```python
from build123d import *

# Parameters (mm, degrees)
F0_W      = 12.7
F0_H      = 50.8
F1_DEPTH  = 11.0998
F3_DEPTH  = 5.08
F3_TAPER  = 3
F4_W      = 12.7
F4_H      = 19.05
F5_DEPTH  = 47.0916
F6_W      = 6.35
F6_H      = 19.05
F7_DEPTH  = 126.7968
F8_W      = 12.7
F8_H      = 19.05
F9_DEPTH  = 40.7416
F10_W     = 12.7
F10_H     = 50.8
F11_DEPTH = 11.0998
F13_DEPTH = 5.334
F13_TAPER = 3
F14_W     = 25.4
F14_H     = 76.2
F15_DEPTH = 12.7
F16_W     = 25.4
F16_H     = 76.2
F17_DEPTH = 12.7
F18_R     = 3.96875
F19_DEPTH = 139.4978
F20_R     = 2.54
F21_DEPTH = 16.4348001
F22_R     = 2.54
F23_DEPTH = 58.1924
F24_R     = 3.81
F25_DEPTH = 45.4914
F26_R     = 6.35


with BuildPart() as f1:
    # F0 (on Right) → F1 (new body)
    with BuildSketch(Plane.YZ):
        with Locations((6.35, 25.4)):
            Rectangle(F0_W, F0_H)
    extrude(amount=F1_DEPTH)

    # F2 (on face) → F3 (join)
    with BuildSketch(Plane.YZ.offset(11.0998)):
        Polygon((4.191, 34.3605023065), (8.509, 34.3605023065), (10.668, 38.1), (8.509, 41.8394976935), (4.191, 41.8394976935), (2.032, 38.1), align=None)
    extrude(amount=F3_DEPTH, taper=F3_TAPER)

    # F4 (on face) → F5 (join)
    with BuildSketch(Plane(origin=(0, 0, 0), x_dir=(0, -1, 0), z_dir=(-1, 0, 0))):
        with Locations((-6.35, 9.525)):
            Rectangle(F4_W, F4_H)
    extrude(amount=F5_DEPTH)

    # F6 (on face) → F7 (join)
    with BuildSketch(Plane.XZ):
        with Locations((-43.9166, 9.525)):
            Rectangle(F6_W, F6_H)
    extrude(amount=F7_DEPTH)

    # F8 (on face) → F9 (join, through all)
    with BuildSketch(Plane.YZ.offset(-40.7416)):
        with Locations((-120.4468, 9.525)):
            Rectangle(F8_W, F8_H)
    extrude(amount=F9_DEPTH)

    # F10 (on face) → F11 (join)
    with BuildSketch(Plane.YZ):
        with Locations((-120.4468, 25.4)):
            Rectangle(F10_W, F10_H)
    extrude(amount=F11_DEPTH)

    # F12 (on face) → F13 (join)
    with BuildSketch(Plane.YZ.offset(11.0998)):
        Polygon((-118.2878, 41.8394976935), (-122.6058, 41.8394976935), (-124.7648, 38.1), (-122.6058, 34.3605023065), (-118.2878, 34.3605023065), (-116.1288, 38.1), align=None)
    extrude(amount=F13_DEPTH, taper=F13_TAPER)

    # F14 (on face) → F15 (join, through all)
    with BuildSketch(Plane(origin=(0, 12.7, 0), x_dir=(-1, 0, 0), z_dir=(0, 1, 0))):
        with Locations((34.3916, 38.1)):
            Rectangle(F14_W, F14_H)
    extrude(amount=-F15_DEPTH)

    # F16 (on face) → F17 (join, through all)
    with BuildSketch(Plane.XZ.offset(126.7968)):
        with Locations((-34.3916, 38.1)):
            Rectangle(F16_W, F16_H)
    extrude(amount=-F17_DEPTH)

    # F18 (on face) → F19 (cut, through all)
    with BuildSketch(Plane(origin=(0, 12.7, 0), x_dir=(-1, 0, 0), z_dir=(0, 1, 0))):
        with Locations((28.4226, 20.9296)):
            Circle(F18_R)
        with Locations((28.4226, 55.3466)):
            Circle(F18_R)
    extrude(amount=-F19_DEPTH, mode=Mode.SUBTRACT)

    # F20 (on face) → F21 (cut, through all)
    with BuildSketch(Plane(origin=(0, 0, 0), x_dir=(0, -1, 0), z_dir=(-1, 0, 0))):
        with Locations((-6.35, 6.35)):
            Circle(F20_R)
    extrude(amount=-F21_DEPTH, mode=Mode.SUBTRACT)

    # F22 (on face) → F23 (cut, through all)
    with BuildSketch(Plane.YZ.offset(11.0998)):
        with Locations((-120.4468, 6.35)):
            Circle(F22_R)
        with Locations((6.35, 6.35)):
            Circle(F22_R)
    extrude(amount=-F23_DEPTH, mode=Mode.SUBTRACT)

    # F24 (on face) → F25 (cut, through all)
    with BuildSketch(Plane(origin=(-47.0916, 0, 0), x_dir=(0, -1, 0), z_dir=(-1, 0, 0))):
        with Locations((120.4468, 6.35)):
            Circle(F24_R)
        with Locations((-6.35, 6.35)):
            Circle(F24_R)
    extrude(amount=-F25_DEPTH, mode=Mode.SUBTRACT)

    # F26
    f26_edges = [f1.edges().sort_by_distance(p)[0] for p in [
        (0, 6.35, 19.05),
        (-21.6916, 6.35, 19.05),
        (-21.6916, -120.4468, 19.05),
        (0, -120.4468, 19.05),
        (-47.0916, 0, 47.625),
        (-21.6916, 6.35, 76.2),
        (-47.0916, -120.4468, 76.2),
        (-21.6916, -120.4468, 76.2),
    ]]
    fillet(f26_edges, radius=F26_R)


solid = f1.part
```
Verification items for the finished model (mm, model axes). A direction names the side the tool comes from. Give positions to 0.01 mm unless a question says otherwise; leave off trailing zeros. Order: outer loops, then holes, each group sorted by start corner. A loop starts at its lowest first (then second) coordinate and runs counter-clockwise, first axis right, second up. Notation, with made-up numbers: (68, 57) -> (84, 57) arc R8 cw to (84, 63) -> close; hole circle Ø1 at (-8, 17.25). An arc over 180 degrees is marked (long way). One line per item, written item: value.
(1) Sectioned sample at C-C on x = 2. Record the cut outline in (y, z), then the cut area to 3 significant figures.
Final values:
outline: (-126.8, 0) -> (-114.1, 0) -> (-114.1, 50.8) -> (-126.8, 50.8) -> close; (0, 0) -> (12.7, 0) -> (12.7, 50.8) -> (0, 50.8) -> close; hole circle Ø5.08 at (-120.45, 6.35); hole circle Ø5.08 at (6.35, 6.35)
area: 1,250 mm^2
(2) Sectioned sample at A-A on x = -35. Record the cut outline in (y, z), then the cut area to 3 significant figures.
Final values:
outline: (-126.8, 0) -> (-114.1, 0) -> (-114.1, 76.2) -> (-126.8, 76.2) -> close; (0, 0) -> (12.7, 0) -> (12.7, 76.2) -> (0, 76.2) -> close; hole circle Ø7.62 at (-120.45, 6.35); hole circle Ø7.62 at (6.35, 6.35)
area: 1,840 mm^2
(3) Draft check along X on faces 6 (the face through (-34, -121, 76.2)), 7 (the face through (16.434, -120, 38)), 8 (the face through (-21.692, 6, 47)). Enter one of: pulls with the +X half, pulls with the -X half, needs draft (parallel to the pull), parting line crosses it, or undercut.
Final values:
face 6: needs draft
face 7: pulls with the +X half
face 8: undercut
(4) Sectioned sample at D-D on y = -100. Record the cut outline in (x, z), then the cut area to 3 significant figures.
Final values:
outline: (-47.09, 0) -> (-40.74, 0) -> (-40.74, 19.05) -> (-47.09, 19.05) -> close
area: 121 mm^2
(5) Scan lines: line 1 along Y through (x, z) = (-10, 19); line 2 along X through (y, z) = (-23, 5); line 3 along X through (y, z) = (1, 70). Record each from-to range of solid material in increasing order. Write a range as [from, to].
Final values:
line 1: [-126.8, -114.1], [0, 12.7]
line 2: [-47.09, -40.74]
line 3: [-44.16, -21.69]
(6) Tool access check on faces 1 (the face through (0, -121, 38)), 2 (the face through (5, -121, 50.8)), 3 (the face through (-40.742, -56, 9)), 4 (the face through (-45.28, 1.91, 48.03)), 5 (the face through (-45.28, -120.36, 74.29)). Record the directions out of +Z, -Z, +X, -X, +Y, -Y that give a thin tool (end or side, any length) a straight path to the whole face; none if there is none.
Final values:
face 1: +Z, +Y, -Y
face 2: +Z, +X, +Y, -Y
face 3: +Z, -Z, +X
face 4: +Z, -X
face 5: +Z, -X, -Y
(7) Gauge pin test, flat ends, axial feed: pin 1 (3.5 mm diameter, centred on x = 7.5, y = -121.5, fed in from +Z); pin 2 (5.5 mm diameter, centred on y = -81, z = 11, fed in from +X); pin 3 (3.5 mm diameter, centred on y = 5.5, z = 39, fed in from +X); pin 4 (9 mm diameter, centred on x = -28.42, z = 20.93, fed in from +Y). Record the tip position at first contact, or that the pin passes through.
Final values:
pin 1: z = 50.8
pin 2: x = -40.74
pin 3: x = 16.18
pin 4: y = 12.7
(8) Sectioned sample at B-B on z = 65.5. Record the cut outline in (x, y), then the cut area to 3 significant figures.
Final values:
outline: (-47.09, -126.8) -> (-21.69, -126.8) -> (-21.69, -114.1) -> (-47.09, -114.1) -> close; (-47.09, 6.35) arc R6.35 ccw to (-40.74, 0) -> (-21.69, 0) -> (-21.69, 12.7) -> (-47.09, 12.7) -> close
area: 637 mm^2
